Input: part model. Units: mm. Frame: model coordinates. A direction names the side the tool comes from. Coordinates: 2 decimals unless noted, no trailing zeros. Loops run counter-clockwise (first coordinate to the right, second up) from the corner with the lowest first, then second, coordinate; pieces in that order, holes last. Notation, with made-up numbers: M 68.5,44.5 L 107.5,44.5 A19 ccw 107.5,70.5 Z; hole C 55.5,85 d8. An arc over 180 degrees is marked long. Use a Markdown table: item, result. Add a question column.
1. Set-up query: faces 1 (the flat face through (21, -16.5, 0)), 2 (the flat face through (19, 29, 0)), 3 (the flat face through (19, -5, 0)). Return all of +Z, -Z, +X, -X, +Y, -Y with unobstructed straight access to the full face (end or side cutting, diameter ignored); none if empty.
2. Draft query along Y for faces 4 (the cylindrical face through (20.521, -13.235, -0.228)), 5 (the flat face through (10, 6, 0)), 6 (the flat face through (11, 14, -12.25)). Return one class per face: +Y half, -Y half, draft (parallel to the pull), parting line (faces both ways), or undercut.
3. Section C-C on z = -10. Output: boundary loops of the cut face in (x, y).
4. Pin query (flat end, axial travel): pin 1 (5 mm diameter, centred on y = 0.5, z = 3, fed in from -X); pin 2 (7.5 mm diameter, centred on x = 8, z = 5, fed in from -Y); pin 3 (8 mm diameter, centred on x = -9, y = 14.5, fed in from -Z). Return the tip coordinate at first contact, or that it passes through.
5. Line query: L1, parallel to Y at x = 20.4, z = 0; L2, parallel to Z at x = 0, y = 18; L3, parallel to X at y = 21.25, z = 0. Output: solid intervals per line, ascending. Write a range as [from, to].
6. Section A-A on z = 5. Output: boundary loops of the cut face in (x, y).
7. Section B-B on x = -2.5. Output: boundary loops of the cut face in (y, z), then the cut area to 3 significant figures.
8. Section D-D on y = 28. Output: boundary loops of the cut face in (x, z), then the cut area to 3 significant figures.
```python
from build123d import *

# Parameters (mm, degrees)
BOSS_EXTRUDE1_DEPTH = 20
SKETCH2_W           = 24.5
SKETCH2_H           = 16.5
SKETCH2_R           = 1.75
BOSS_EXTRUDE2_DEPTH = 3
FILLET1_R           = 5
SKETCH4_R           = 9.25
BOSS_EXTRUDE4_DEPTH = 6
SKETCH3_R           = 9.25
CUT_EXTRUDE1_DEPTH  = 6


with BuildPart() as part:
    # Sketch1 → Boss-Extrude1 (new body)
    with BuildSketch(Plane(origin=(0, 0, 0), x_dir=(1, 0, 0), z_dir=(0, 1, 0))):
        with BuildLine():
            Line((0, 12.25), (0, 9.25))
            ThreePointArc((0, 9.25), (6.540737726, 6.540737726), (9.25, 0))
            ThreePointArc((9.25, 0), (6.540737726, -6.540737726), (0, -9.25))
            Line((0, -9.25), (0, -12.25))
            Line((0, -12.25), (22, -12.25))
            Line((22, -12.25), (22, 12.25))
            Line((22, 12.25), (0, 12.25))
        make_face()
        with BuildLine():
            ThreePointArc((0, -9.25), (-9.25, 0), (0, 9.25))
            Line((0, 9.25), (0, 12.25))
            ThreePointArc((0, 12.25), (-12.25, 0), (0, -12.25))
            Line((0, -12.25), (0, -9.25))
        make_face()
    extrude(amount=BOSS_EXTRUDE1_DEPTH)

    # Sketch2 → Boss-Extrude2 (add)
    with BuildSketch(Plane(origin=(22, 0, 0), x_dir=(0, 0, -1), z_dir=(1, 0, 0))):
        with Locations((0, 28.25)):
            Rectangle(SKETCH2_W, SKETCH2_H)
        with Locations((0, 31.5)):
            Circle(SKETCH2_R, mode=Mode.SUBTRACT)
        with Locations((0, -8.25)):
            Rectangle(SKETCH2_W, SKETCH2_H)
        with Locations(Location((0, -11.5, 0), (0, 0, 180))):
            Circle(SKETCH2_R, mode=Mode.SUBTRACT)
    extrude(amount=-BOSS_EXTRUDE2_DEPTH)

    # Fillet1
    fillet1_edges = [part.edges().sort_by_distance(p)[0] for p in [
        (20.5, 36.5, 12.25),
        (20.5, 36.5, -12.25),
        (20.5, -16.5, -12.25),
        (20.5, -16.5, 12.25),
    ]]
    fillet(fillet1_edges, radius=FILLET1_R)

    # Sketch4 → Boss-Extrude4 (add)
    with BuildSketch(Plane(origin=(0, 20, 0), x_dir=(1, 0, 0), z_dir=(0, 1, 0))):
        with BuildLine():
            Line((0, -12.25), (19, -12.25))
            Line((19, -12.25), (19, 12.25))
            Line((19, 12.25), (0, 12.25))
            ThreePointArc((0, 12.25), (-12.25, 0), (0, -12.25))
        make_face()
        with Locations(Location((0, 0, 0), (0, 0, 270))):
            Circle(SKETCH4_R, mode=Mode.SUBTRACT)
    extrude(amount=BOSS_EXTRUDE4_DEPTH)

    # Sketch3 → Cut-Extrude1 (cut)
    with BuildSketch(Plane.XZ):
        with BuildLine():
            Line((0, -12.25), (19, -12.25))
            Line((19, -12.25), (19, 12.25))
            Line((19, 12.25), (0, 12.25))
            ThreePointArc((0, 12.25), (-12.25, 0), (0, -12.25))
        make_face()
        with Locations(Location((0, 0, 0), (0, 0, 270))):
            Circle(SKETCH3_R, mode=Mode.SUBTRACT)
    extrude(amount=-CUT_EXTRUDE1_DEPTH, mode=Mode.SUBTRACT)


solid = part.part
```
Answers below:
| question | item | result |
|---|---|---|
| 1 | face 1 | +Z, -Z, +X, -X, -Y |
| 1 | face 2 | +Z, -Z, -X, +Y |
| 1 | face 3 | +Z, -Z, -X, -Y |
| 2 | face 4 | undercut |
| 2 | face 5 | -Y half |
| 2 | face 6 | draft |
| 3 | outline | M -7.08,6 L 19,6 L 19,-15.68 L 22,-15.68 L 22,35.68 L 19,35.68 L 19,26 L -7.08,26 Z |
| 4 | pin 1 | stops at x = 19 |
| 4 | pin 2 | stops at y = 6 |
| 4 | pin 3 | stops at z = -11.18 |
| 5 | L1 | y = [-16.5, -13.25], [-9.75, 29.75], [33.25, 36.5] |
| 5 | L2 | z = [-12.25, -9.25], [9.25, 12.25] |
| 5 | L3 | x = [-12.25, -9.25], [9.25, 22] |
| 6 | outline | M -11.18,6 L -7.78,6 L -7.78,26 L -11.18,26 Z; M 7.78,6 L 19,6 L 19,-16.5 L 22,-16.5 L 22,36.5 L 19,36.5 L 19,26 L 7.78,26 Z |
| 7 | outline | M 6,-11.99 L 26,-11.99 L 26,-8.91 L 6,-8.91 Z; M 6,8.91 L 26,8.91 L 26,11.99 L 6,11.99 Z |
| 7 | area | 123 mm² |
| 8 | outline | M 19,-12.25 L 22,-12.25 L 22,12.25 L 19,12.25 Z |
| 8 | area | 73.5 mm² |
